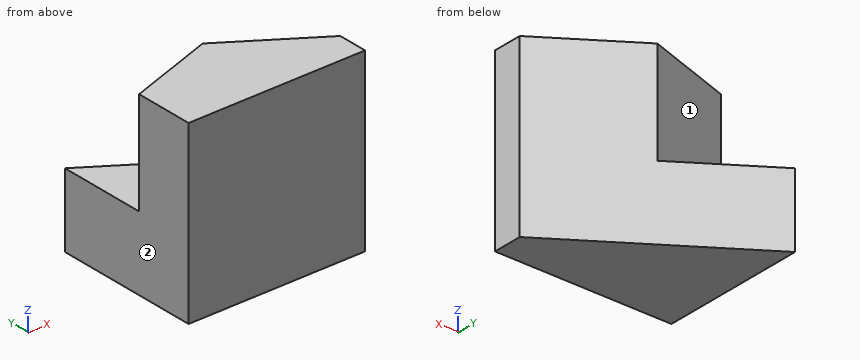
from build123d import *

# Parameters (mm, degrees)
SKETCH1_W           = 6
SKETCH1_H           = 6
BOSS_EXTRUDE1_DEPTH = 5
CUT_EXTRUDE7_DEPTH  = 8
CUT_EXTRUDE8_DEPTH  = 3.5


with BuildPart() as part:
    # Sketch1 → Boss-Extrude1 (new body)
    with BuildSketch(Plane(origin=(0, 0, 0), x_dir=(1, 0, 0), z_dir=(0, 1, 0))):
        Rectangle(SKETCH1_W, SKETCH1_H)
    extrude(amount=BOSS_EXTRUDE1_DEPTH)

    # Sketch10 → Cut-Extrude7 (cut)
    with BuildSketch(Plane.XY.offset(3)):
        Polygon((3, 5), (-3, 5), (3, 1), align=None)
    extrude(amount=-CUT_EXTRUDE7_DEPTH, mode=Mode.SUBTRACT)

    # Sketch11 → Cut-Extrude8 (cut)
    with BuildSketch(Plane.XY.offset(3)):
        Polygon((-3, 5), (-3, 2), (0, 3), align=None)
    extrude(amount=-CUT_EXTRUDE8_DEPTH, mode=Mode.SUBTRACT)


solid = part.part
Work out the finished part from the listing and answer in its coordinate system (mm). Face numbers are marked on the shaded views. A direction names the side the tool comes from. Coordinates: 2 decimals unless noted, no trailing zeros. Loops run counter-clockwise (first coordinate to the right, second up) from the corner with the lowest first, then second, coordinate; pieces in that order, holes last. Notation, with made-up numbers: M 77.5,42 L 101.5,42 A11 cw 101.5,56 Z; hole C 87,27.5 d1. An arc over 180 degrees is marked long. Answer in a Markdown table with one row per item. Add a question column.
1. Find section C-C, the plane x = -0.5. Write down the section's boundary in (y, z), then the cut area to 4 significant figures.
2. Flat-ended cylindrical pins translate along their axes: P1, Ø1.5, axis at x = -2, y = 4, coming from the +Z side; P2, Ø3, axis at x = 1.5, z = 1.5, coming from the -Y side. Find the tip coordinate at first contact, or state that the pin passes through.
3. Find section A-A, the plane y = 2.6. Write down the section's boundary in (x, z), then the cut area to 3 significant figures.
4. Find section D-D, the plane y = 3.8. Write down the section's boundary in (x, z), then the cut area to 3 significant figures.
5. A tool of negligible diameter and unlimited length cuts with its end or side. For the marked faces 1 and 2, from which of +Z, -Z, +X, -X, +Y, -Y can it reach the whole face along a straight path? Write none if from no direction.
6. Find section B-B, the plane z = 2.2. Write down the section's boundary in (x, y).
7. Consider L1, parallel to Z at x = -1.75, y = 2.5; L2, parallel to Y at x = 1.5, z = -2.2; L3, parallel to Y at x = 1.25, z = -1.95. Determine where each line is inside the solid, lowest interval first.
Reported:
| question | item | result |
|---|---|---|
| 1 | outline | M 0,-3 L 3.33,-3 L 3.33,-0.5 L 2.83,-0.5 L 2.83,3 L 0,3 Z |
| 1 | area | 18.25 mm^2 |
| 2 | P1 | stops at z = -0.5 |
| 2 | P2 | stops at y = 0 |
| 3 | outline | M -3,-3 L 0.6,-3 L 0.6,3 L -1.2,3 L -1.2,-0.5 L -3,-0.5 Z |
| 3 | area | 15.3 mm^2 |
| 4 | outline | M -3,-3 L -1.2,-3 L -1.2,-0.5 L -3,-0.5 Z |
| 4 | area | 4.50 mm^2 |
| 5 | face 1 | +Z, -X, +Y |
| 5 | face 2 | +Z, -Z, -X, +Y, -Y |
| 6 | outline | M -3,0 L 3,0 L 3,1 L 0,3 L -3,2 Z |
| 7 | L1 | z = -3 to -0.5 |
| 7 | L2 | y = 0 to 2 |
| 7 | L3 | y = 0 to 2.17 |
